The model under review builds one solid part; all positions refer to its coordinate system, in mm. A direction names the side the tool comes from. Round coordinates to 2 decimals unless told otherwise and drop trailing zeros. Order: outer loops, then holes, each group sorted by start corner. A loop starts at its lowest first (then second) coordinate and runs counter-clockwise, first axis right, second up. Notation, with made-up numbers: M -19.75,-40 L -1.75,-40 A20 ccw -1.75,-4 Z; hole C 6.5,20.5 d11. An arc over 180 degrees is marked long. Answer as a JSON object with one key per item and string values. Group by question number.
1) To check wall thickness, follow line 1 (Y direction, x = 0, z = 2.1) (1 decimal); line 2 (Y direction, x = 0, z = 3.3); line 3 (Z direction, x = 10.5, y = 8). State the ranges of each line that lie inside material, in increasing order.
2) Consider section A-A, the plane x = 0. Count the separate pieces of the cut face and the enclosed holes in it, then the cut area to 3 significant figures.
3) Insertion check: pin 1 Ø12 at (y, z) = (-2.5, 15) entering from +X; pin 2 Ø2 at (x, y) = (-6, 1) entering from +Z; pin 3 Ø5 at (x, y) = (6.5, -5.5) entering from -Z; pin 4 Ø4 at (x, y) = (-7, -3.5) entering from +Z. Each pin has a flat end and moves straight along its axis. Give the tip position at first contact, or say it passes through.
4) For faces 1 (the flat face through (0, -6, 2.85)), 2 (the flat face through (-10, 7.275, -1)), 3 (the cylindrical face through (5.102, -7.082, 28.407)), list the 3-axis set-ups (+Z, -Z, +X, -X, +Y, -Y) from which the entire face can be reached by the end or side of a thin tool; tool diameter is ignored.
5) Consider section D-D, the plane z = 6.5. Write out the cut boundary in (x, y), then the cut area to 3 significant figures.
6) Consider section C-C, the plane x = 7.25. Write out the cut boundary in (y, z), then the cut area to 3 significant figures.
7) The part is to be moulded in two halves that separate along X. For faces 4 (the flat face through (-7, -3.5, 30)), 5 (the cylindrical face through (-0.274, 4.365, 1.506)), 6 (the flat face through (0, 6, 2.85)), 7 (the cylindrical face through (14.75, 9.57, 28.61)), say which applies: +X half, -X half, draft (parallel to the pull), parting line (faces both ways), or undercut.
```python
from build123d import *

# Parameters (mm, degrees)
SKETCH_1_R          = 3.2375
EXTRUDE_1_DEPTH     = 5
SKETCH_2_R          = 1.265
CUT_EXTRUDE_1_DEPTH = 2.85
CHAMFER_1_SIZE      = 0.2
SKETCH_5_W          = 1.72
SKETCH_5_H          = 14.55
EXTRUDE_2_DEPTH     = 1.55
CHAMFER_2_SIZE      = 0.2
FILLET_1_R          = 0.15
SKETCH_6_W          = 4.8
SKETCH_6_H          = 20
EXTRUDE_3_DEPTH     = 31
EXTRUDE_START       = 31
SKETCH_7_W          = 25.9
SKETCH_7_H          = 20
EXTRUDE_4_DEPTH     = 4.92
CUT_EXTRUDE_START   = 26.08
SKETCH_8_R          = 1.52
CUT_EXTRUDE_2_DEPTH = 4.92
CHAMFER_3_SIZE      = 0.2
CUT_EXTRUDE_START_2 = 31
SKETCH_10_W         = 4.38
SKETCH_10_H         = 20
CUT_EXTRUDE_3_DEPTH = 31
FILLET_2_R          = 1.5
CUT_EXTRUDE_4_DEPTH = 2
SKETCH_13_W         = 3.2
SKETCH_13_H         = 20
EXTRUDE_5_DEPTH     = 5
CHAMFER_5_SIZE      = 3
CUT_EXTRUDE_START_3 = 5
CUT_EXTRUDE_5_DEPTH = 7
CHAMFER_7_SIZE      = 1.3
CHAMFER_8_SIZE      = 0.2


with BuildPart() as part:
    # 草图1 → 凸台-拉伸1 (new body)
    with BuildSketch(Plane.XY):
        Polygon((13.5775, 0), (13.5775, 10), (-10.48, 10), (-10.48, 0), (-10.48, -10), (13.5775, -10), align=None)
        Circle(SKETCH_1_R, mode=Mode.SUBTRACT)
    extrude(amount=EXTRUDE_1_DEPTH)

    # 草图2 → 切除-拉伸1 (cut)
    with BuildSketch(Plane.XY):
        with Locations((0, 5.6)):
            Circle(SKETCH_2_R)
        with Locations((0, -5.6)):
            Circle(SKETCH_2_R)
    extrude(amount=CUT_EXTRUDE_1_DEPTH, mode=Mode.SUBTRACT)

    # 倒角1
    chamfer_1_edges = [part.edges().sort_by_distance(p)[0] for p in [
        (-1.265, 5.6, 0),
        (-1.265, -5.6, 0),
    ]]
    chamfer(chamfer_1_edges, length=CHAMFER_1_SIZE)

    # 草图5 → 凸台-拉伸2 (add)
    with BuildSketch(Plane.XY):
        with Locations((-9.62, 0)):
            Rectangle(SKETCH_5_W, SKETCH_5_H)
    extrude(amount=-EXTRUDE_2_DEPTH)

    # 倒角2
    chamfer_2_edges = [part.edges().sort_by_distance(p)[0] for p in [
        (-10.48, 0, -1.55),
        (-9.62, 7.275, -1.55),
        (-8.76, 0, -1.55),
        (-9.62, -7.275, -1.55),
    ]]
    chamfer(chamfer_2_edges, length=CHAMFER_2_SIZE)

    # 圆角1
    fillet_1_edges = [part.edges().sort_by_distance(p)[0] for p in [
        (-8.76, -7.275, -0.675),
        (-8.76, 7.275, -0.675),
        (-10.48, -7.275, -0.675),
        (-10.48, 7.275, -0.675),
    ]]
    fillet(fillet_1_edges, radius=FILLET_1_R)

    # 草图6 → 凸台-拉伸3 (add)
    with BuildSketch(Plane.XY):
        with Locations((-8.08, 0)):
            Rectangle(SKETCH_6_W, SKETCH_6_H)
    extrude(amount=EXTRUDE_3_DEPTH)

    # 草图7 → 凸台-拉伸4 (add)
    with BuildSketch(Plane.XY.offset(EXTRUDE_START)):
        with Locations((6.6275, 0)):
            Rectangle(SKETCH_7_W, SKETCH_7_H)
    extrude(amount=-EXTRUDE_4_DEPTH)

    # 草图8 → 切除-拉伸2 (cut)
    with BuildSketch(Plane.XY.offset(CUT_EXTRUDE_START)):
        with Locations((3.6975, 6.5)):
            Circle(SKETCH_8_R)
        with Locations((11.6975, 6.5)):
            Circle(SKETCH_8_R)
        with Locations((11.6975, -6.5)):
            Circle(SKETCH_8_R)
        with Locations((3.6975, -6.5)):
            Circle(SKETCH_8_R)
    extrude(amount=CUT_EXTRUDE_2_DEPTH, mode=Mode.SUBTRACT)

    # 倒角3
    chamfer_3_edges = [part.edges().sort_by_distance(p)[0] for p in [
        (2.1775, -6.5, 31),
        (10.1775, -6.5, 31),
        (10.1775, 6.5, 31),
        (2.1775, 6.5, 31),
    ]]
    chamfer(chamfer_3_edges, length=CHAMFER_3_SIZE)

    # 草图10 → 切除-拉伸3 (cut)
    with BuildSketch(Plane.XY.offset(CUT_EXTRUDE_START_2)):
        with Locations((17.3875, 0)):
            Rectangle(SKETCH_10_W, SKETCH_10_H)
    extrude(amount=-CUT_EXTRUDE_3_DEPTH, mode=Mode.SUBTRACT)

    # 圆角2
    fillet_2_edges = [part.edges().sort_by_distance(p)[0] for p in [
        (15.1975, -10, 28.54),
        (15.1975, 10, 28.54),
    ]]
    fillet(fillet_2_edges, radius=FILLET_2_R)

    # 草图11 → 切除-拉伸4 (cut)
    with BuildSketch(Plane.XY.offset(CUT_EXTRUDE_START_2)):
        with BuildLine():
            Line((-4.48, 3.5), (-10.48, 3.5))
            Line((-10.48, 3.5), (-10.48, -3.5))
            Line((-10.48, -3.5), (-4.48, -3.5))
            ThreePointArc((-4.48, -3.5), (-0.98, 0), (-4.48, 3.5))
        make_face()
    extrude(amount=-CUT_EXTRUDE_4_DEPTH, mode=Mode.SUBTRACT)

    # 草图13 → 凸台-拉伸5 (add)
    with BuildSketch(Plane.XY):
        with Locations((10.798987738, 0)):
            Rectangle(SKETCH_13_W, SKETCH_13_H)
    extrude(amount=EXTRUDE_5_DEPTH)

    # 倒角5
    chamfer_5_edges = [part.edges().sort_by_distance(p)[0] for p in [
        (13.5775, 0, 5),
    ]]
    chamfer(chamfer_5_edges, length=CHAMFER_5_SIZE)

    # 草图14 → 切除-拉伸5 (cut)
    with BuildSketch(Plane.XY.offset(CUT_EXTRUDE_START_3)):
        with BuildLine():
            Line((-5.284271247, 10), (-5.284271247, -10))
            ThreePointArc((-5.284271247, -10), (-7, 0), (-5.284271247, 10))
        make_face()
    extrude(amount=CUT_EXTRUDE_5_DEPTH, mode=Mode.SUBTRACT)

    # 倒角7
    chamfer_7_edges = [part.edges().sort_by_distance(p)[0] for p in [
        (-5.68, 0, 12),
    ]]
    chamfer(chamfer_7_edges, length=CHAMFER_7_SIZE)

    # 倒角8
    chamfer_8_edges = [part.edges().sort_by_distance(p)[0] for p in [
        (2.44875, -10, 5),
        (-5.68, -10, 15.54),
        (-5.68, 10, 15.54),
        (4.00875, 10, 26.08),
        (4.00875, -10, 26.08),
        (15.1975, 0, 26.08),
        (14.758160172, 9.560660172, 26.08),
        (14.758160172, -9.560660172, 26.08),
        (-7.48, 3.5, 31),
        (-10.48, 3.5, 30),
        (-7.48, -3.5, 31),
        (-10.48, -3.5, 30),
        (-10.48, 0, 29),
        (-0.98, 0, 31),
        (2.44875, 10, 5),
        (13.5775, 10, 1),
        (12.0775, 10, 3.5),
        (13.5775, -10, 1),
        (12.0775, -10, 3.5),
        (1.54875, -10, 0),
        (1.54875, 10, 0),
        (13.5775, 0, 0),
    ]]
    chamfer(chamfer_8_edges, length=CHAMFER_8_SIZE)


solid = part.part
```
Results list:
{
 "1": {"line 1": "-10 to -6.9, -4.3 to -3.2, 3.2 to 4.3, 6.9 to 10", "line 2": "-10 to -3.24, 3.24 to 10", "line 3": "0 to 5, 26.08 to 31"},
 "2": {"separate pieces": "3", "enclosed holes": "0", "area": "151 mm^2"},
 "3": {"pin 1": "x = -5.68", "pin 2": "z = 29", "pin 3": "z = 0", "pin 4": "z = 31"},
 "4": {"face 1": "-Z", "face 2": "-Z, +X, -X, +Y", "face 3": "+Z"},
 "5": {"outline": "M -10.48,-10 L -5.88,-10 L -5.68,-9.8 L -5.68,-8.8 A30 cw -5.68,8.8 L -5.68,9.8 L -5.88,10 L -10.48,10 Z", "area": "80.4 mm^2"},
 "6": {"outline": "M -10,0.2 L -9.8,0 L 9.8,0 L 10,0.2 L 10,4.8 L 9.8,5 L -9.8,5 L -10,4.8 Z; M -10,26.28 L -9.8,26.08 L 9.8,26.08 L 10,26.28 L 10,31 L -10,31 Z", "area": "198 mm^2"},
 "7": {"face 4": "draft", "face 5": "undercut", "face 6": "undercut", "face 7": "+X half"}
}
